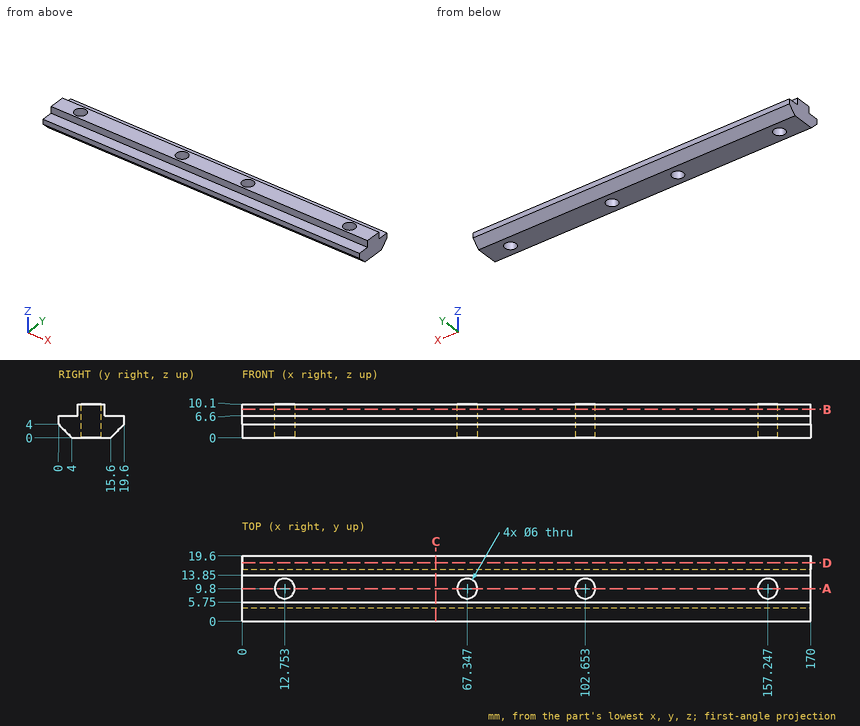
Part print with two shaded views. Sizes in mm from the minimum x, y, z corner. Coordinates: 2 decimals unless noted, no trailing zeros. Write each loop counter-clockwise with the first axis right and the second up, starting at its lowest first coordinate (ties: lowest second). Pieces come first, ordered by that corner, then holes.
(1) Drill centre lines: line 1 (Y direction, x = 70, z = 7.5); line 2 (Y direction, x = 49.5, z = 8.5); line 3 (Y direction, x = 11.5, z = 1) (1 decimal). Where is each one in solid material? Low to high.
(2) Cut at D-D on y = 17.5. List the corners of the cut face in (x, z), and give its area (3 significant figures).
(3) Cut at B-B on z = 8.5. List the corners of the cut face in (x, y).
(4) Pin check, flat tips, straight feed: pin 1 Ø1.7 at (x, y) = (72.5, 16) entering from +Z; pin 2 Ø1 at (x, z) = (57.5, 1) entering from -Y. Stop position of each tip, or through.
(5) Cut at A-A on y = 9.8. List the corners of the cut face in (x, z).
(6) Cut at C-C on x = 58. List the corners of the cut face in (y, z), and give its area (3 significant figures).
Working result:
1. line 1: y = 5.75 to 8.4, 11.2 to 13.85
1. line 2: y = 5.75 to 13.85
1. line 3: y = 3 to 7.1, 12.5 to 16.6
2. outline: (0, 1.9) - (170, 1.9) - (170, 6.6) - (0, 6.6) - close
2. area: 799 mm2
3. outline: (0, 5.75) - (170, 5.75) - (170, 13.85) - (0, 13.85) - close; hole circle Ø6 at (12.75, 9.8); hole circle Ø6 at (67.35, 9.8); hole circle Ø6 at (102.65, 9.8); hole circle Ø6 at (157.25, 9.8)
4. pin 1: stops at z = 6.6
4. pin 2: stops at y = 2.5
5. outline: (0, 0) - (9.75, 0) - (9.75, 10.1) - (0, 10.1) - close; (15.75, 0) - (64.35, 0) - (64.35, 10.1) - (15.75, 10.1) - close; (70.35, 0) - (99.65, 0) - (99.65, 10.1) - (70.35, 10.1) - close; (105.65, 0) - (154.25, 0) - (154.25, 10.1) - (105.65, 10.1) - close; (160.25, 0) - (170, 0) - (170, 10.1) - (160.25, 10.1) - close
6. outline: (0, 4) - (4, 0) - (15.6, 0) - (19.6, 4) - (19.6, 6.6) - (13.85, 6.6) - (13.85, 10.1) - (5.75, 10.1) - (5.75, 6.6) - (0, 6.6) - close
6. area: 142 mm2
